from build123d import *

# Parameters (mm, degrees)
SKETCH_1_R      = 5.1
SKETCH_1_R_2    = 7.5
EXTRUDE_1_DEPTH = 5


with BuildPart() as part:
    # 草图1 → 凸台-拉伸1 (new body)
    with BuildSketch(Plane(origin=(0, 0, 0), x_dir=(1, 0, 0), z_dir=(0, 1, 0))):
        with BuildLine():
            Line((5, 0), (22, 0))
            ThreePointArc((22, 0), (23.414213562, -0.585786438), (24, -2))
            Line((24, -2), (24, -3))
            ThreePointArc((24, -3), (24.878679656, -5.121320344), (27, -6))
            Line((27, -6), (34, -6))
            Line((34, -6), (34, 4))
            Line((34, 4), (29, 4))
            Line((29, 4), (29, 14))
            Line((29, 14), (34, 14))
            Line((34, 14), (34, 42))
            Line((34, 42), (29, 42))
            Line((29, 42), (29, 52))
            Line((29, 52), (34, 52))
            Line((34, 52), (34, 62))
            Line((34, 62), (27, 62))
            ThreePointArc((27, 62), (24.878679656, 61.121320344), (24, 59))
            Line((24, 59), (24, 58))
            ThreePointArc((24, 58), (23.414213562, 56.585786438), (22, 56))
            Line((22, 56), (5, 56))
            ThreePointArc((5, 56), (1.464466094, 54.535533906), (0, 51))
            Line((0, 51), (0, 5))
            ThreePointArc((0, 5), (1.464466094, 1.464466094), (5, 0))
        make_face()
        with Locations(Location((12, 44, 0), (0, 0, 270))):
            Circle(SKETCH_1_R, mode=Mode.SUBTRACT)
        with Locations(Location((12, 12, 0), (0, 0, 270))):
            Circle(SKETCH_1_R_2, mode=Mode.SUBTRACT)
        with BuildLine():
            ThreePointArc((7.25, 52.227241336), (5.282485579, 50.717514421), (3.772758664, 48.75))
            ThreePointArc((3.772758664, 48.75), (4.32179677, 46.700961894), (6.370834875, 47.25))
            ThreePointArc((6.370834875, 47.25), (7.403805922, 48.596194078), (8.75, 49.629165125))
            ThreePointArc((8.75, 49.629165125), (9.299038106, 51.67820323), (7.25, 52.227241336))
        make_face(mode=Mode.SUBTRACT)
        with BuildLine():
            ThreePointArc((20.227241336, 48.75), (18.717514421, 50.717514421), (16.75, 52.227241336))
            ThreePointArc((16.75, 52.227241336), (14.700961894, 51.67820323), (15.25, 49.629165125))
            ThreePointArc((15.25, 49.629165125), (16.596194078, 48.596194078), (17.629165125, 47.25))
            ThreePointArc((17.629165125, 47.25), (19.67820323, 46.700961894), (20.227241336, 48.75))
        make_face(mode=Mode.SUBTRACT)
        with BuildLine():
            ThreePointArc((16.75, 35.772758664), (18.717514421, 37.282485579), (20.227241336, 39.25))
            ThreePointArc((20.227241336, 39.25), (19.67820323, 41.299038106), (17.629165125, 40.75))
            ThreePointArc((17.629165125, 40.75), (16.596194078, 39.403805922), (15.25, 38.370834875))
            ThreePointArc((15.25, 38.370834875), (14.700961894, 36.32179677), (16.75, 35.772758664))
        make_face(mode=Mode.SUBTRACT)
        with BuildLine():
            ThreePointArc((3.772758664, 39.25), (5.282485579, 37.282485579), (7.25, 35.772758664))
            ThreePointArc((7.25, 35.772758664), (9.299038106, 36.32179677), (8.75, 38.370834875))
            ThreePointArc((8.75, 38.370834875), (7.403805922, 39.403805922), (6.370834875, 40.75))
            ThreePointArc((6.370834875, 40.75), (4.32179677, 41.299038106), (3.772758664, 39.25))
        make_face(mode=Mode.SUBTRACT)
    extrude(amount=EXTRUDE_1_DEPTH)


solid = part.part
Design review of the part built by this model. Coordinates are the model's own, in mm. A direction names the side the tool comes from. Round coordinates to 2 decimals unless told otherwise and drop trailing zeros. Order: outer loops, then holes, each group sorted by start corner. A loop starts at its lowest first (then second) coordinate and runs counter-clockwise, first axis right, second up.
1) Consider section B-B (x = 8). State the section outline as (y, z) points.
The answers:
outline: (0, -56) - (5, -56) - (5, -52.43) - (0, -52.43) - close; (0, -49.12) - (5, -49.12) - (5, -47.16) - (0, -47.16) - close; (0, -40.84) - (5, -40.84) - (5, -38.88) - (0, -38.88) - close; (0, -35.57) - (5, -35.57) - (5, -18.34) - (0, -18.34) - close; (0, -5.66) - (5, -5.66) - (5, 0) - (0, 0) - close
2) Consider section D-D (z = -44). State the section outline as (x, y) points.
The answers:
outline: (0, 0) - (6.9, 0) - (6.9, 5) - (0, 5) - close; (17.1, 0) - (29, 0) - (29, 5) - (17.1, 5) - close
3) Consider section C-C (y = 1.5). Count the separate pieces of the cut face and the enclosed holes in it, plus the area to 3 significant figures.
The answers:
separate pieces: 1
enclosed holes: 6
area: 1,570 mm2
4) Consider section A-A (z = -12). State the section outline as (x, y) points.
The answers:
outline: (0, 0) - (4.5, 0) - (4.5, 5) - (0, 5) - close; (19.5, 0) - (29, 0) - (29, 5) - (19.5, 5) - close
5) For L1, parallel to X at y = 2.9, z = -44; L2, parallel to X at y = 2.45, z = -12; L3, parallel to Z at x = 9, y = 4.65, list the stretches that pass through material, from the lowest coordinate up.
The answers:
L1: x = 0 to 6.9, 17.1 to 29
L2: x = 0 to 4.5, 19.5 to 29
L3: z = -56 to -52.05, -49.81 to -48.12, -39.88 to -38.19, -35.95 to -18.87, -5.13 to 0
6) Machinability: for faces 4 (the flat face through (29, 2, -9)), 5 (the cylindrical face through (16.61, 2.46, -39.42)), 6 (the cylindrical face through (1, 2, -2)), which of the approach directions +Z, -Z, +X, -X, +Y, -Y give a long, thin tool a straight path to every point of the face, cutting with its end or side? Answer none if there is none.
The answers:
face 4: +X, +Y, -Y
face 5: +Y, -Y
face 6: +Z, -X, +Y, -Y
7) Draft analysis for pull direction X (two halves, no side actions). For faces 1 (the cylindrical face through (4.68, 2.46, -13.63)), 2 (the flat face through (0, 2, -28)), 3 (the flat face through (31, 2, -52)), state which applies: released by +X, released by -X, zero draft, split by the parting line, or undercut.
The answers:
face 1: undercut
face 2: released by -X
face 3: zero draft
8) Clearance check with flat-ended pins moving along their axes: pin 1 Ø2 at (y, z) = (3.5, -42.5) entering from +X; pin 2 Ø1 at (x, z) = (11, -6) entering from +Y; pin 3 Ø0.5 at (y, z) = (2, -58.5) entering from -X; pin 4 Ø2.5 at (y, z) = (3, -48) entering from +X. State where each tip first meets the part, or that it passes through.
The answers:
pin 1: stops at x = 34
pin 2: passes through
pin 3: stops at x = 24
pin 4: stops at x = 29
